Can you work these out from the model? Positions are in its coordinate system, mm. Face numbers are marked on the shaded views. A direction names the side the tool comes from. Give positions to 0.01 mm unless a question says otherwise; leave off trailing zeros. Order: outer loops, then holes, each group sorted by start corner. A loop starts at its lowest first (then second) coordinate and runs counter-clockwise, first axis right, second up. Notation, with made-up numbers: (32, -32) - (62, -32) arc R11 cw to (62, -28) - close; hole circle Ø4 at (58, -7). An arc over 180 degrees is marked (long way). Answer as a JSON object with one key per item and string values.
```python
from build123d import *

# Parameters (mm, degrees)
F0_W     = 84.4102278352
F0_H     = 68.1378934532
F0_R     = 12.3215660832
F1_DEPTH = 30.734
F2_R     = 13.2353706436
F3_DEPTH = 96.012
F2_R_2   = 9.0233824653
F4_DEPTH = 53.34
F2_R_3   = 4.6999449214
F5_DEPTH = 26.416


with BuildPart() as f1:
    # F0 (on Front) → F1 (new body)
    with BuildSketch(Plane.XZ):
        with Locations((0.754147768, -7.0776222274)):
            Rectangle(F0_W, F0_H)
        Circle(F0_R, mode=Mode.SUBTRACT)
    extrude(amount=F1_DEPTH)

    # F2 (on face) → F3 (join)
    with BuildSketch(Plane.XY.offset(26.9913244992)):
        with Locations((-12.7083817497, -14.5293129608)):
            Circle(F2_R)
    extrude(amount=F3_DEPTH)

    # F2 (on face) → F4 (join)
    with BuildSketch(Plane.XY.offset(26.9913244992)):
        with Locations((9.9861975759, -14.3468007445)):
            Circle(F2_R_2)
    extrude(amount=F4_DEPTH)

    # F2 (on face) → F5 (join)
    with BuildSketch(Plane.XY.offset(26.9913244992)):
        with Locations((-34.5160663128, -12.256086804)):
            Circle(F2_R_3)
    extrude(amount=F5_DEPTH)


solid = f1.part
```
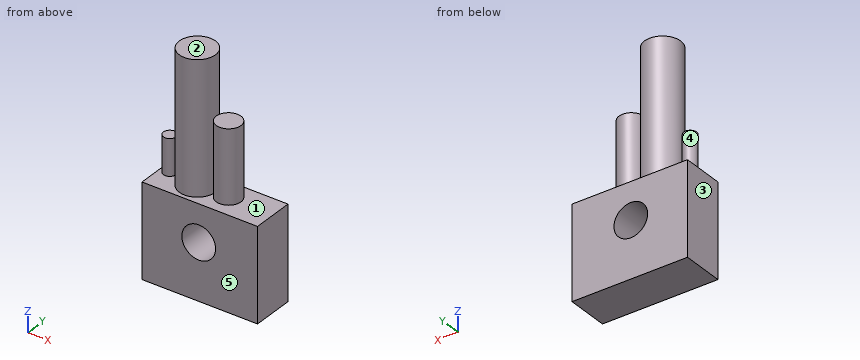
Q1. I'm going to push flat-ended pins straight in: pin 1 Ø12 at (x, y) = (16, -20) entering from +Z; pin 2 Ø10.5 at (x, y) = (-33.5, -13) entering from +Z; pin 3 Ø3 at (x, z) = (-3, 97) entering from -Y. Where does each tip first touch, or does it pass through?
Recorded:
{"pin 1": "stops at z = 80.33", "pin 2": "stops at z = 53.41", "pin 3": "stops at y = -24.91"}
Q2. I need wall thicknesses on L1, parallel to Z at x = 0, y = -10; L2, parallel to Z at x = 0, y = -11; L3, parallel to Z at x = -28, y = -22.5. Which ranges of each line are inside material? Lowest first, please.
Recorded:
{"L1": "z = -41.15 to -12.32, 12.32 to 26.99", "L2": "z = -41.15 to -12.32, 12.32 to 123", "L3": "z = -41.15 to 26.99"}
Q3. Which directions (+Z, -Z, +X, -X, +Y, -Y) give clear straight access to the entire face, cutting with the end or side of a thin tool? Please do the marked faces 1 and 2.
Recorded:
{"face 1": "+Z", "face 2": "+Z, +X, -X, +Y, -Y"}
Q4. If we section it at D-D, the plane x = 29.5: Please give me the cut outline in (y, z).
Recorded:
{"outline": "(-30.73, -41.15) - (0, -41.15) - (0, 26.99) - (-30.73, 26.99) - close"}
Q5. We'd pull the mould along X, two halves only. Please class the marked faces 3, 4 and 5: released by +X, released by -X, zero draft, split by the parting line, or undercut.
Recorded:
{"face 3": "released by -X", "face 4": "undercut", "face 5": "zero draft"}
Q6. If we section it at C-C, the plane y = -21.5: Please give me the cut outline in (x, z).
Recorded:
{"outline": "(-41.45, -41.15) - (42.96, -41.15) - (42.96, 26.99) - (15.49, 26.99) - (15.49, 80.33) - (4.49, 80.33) - (4.49, 26.99) - (-1.46, 26.99) - (-1.46, 123) - (-23.96, 123) - (-23.96, 26.99) - (-41.45, 26.99) - close; hole circle Ø24.64 at (0, 0)"}
Q7. If we section it at A-A, the plane z = 0: Please give me the cut outline in (x, y), then the cut area to 3 significant figures.
Recorded:
{"outline": "(-41.45, -30.73) - (-12.32, -30.73) - (-12.32, 0) - (-41.45, 0) - close; (12.32, -30.73) - (42.96, -30.73) - (42.96, 0) - (12.32, 0) - close", "area": "1,840 mm^2"}
Q8. If we section it at B-B, the plane x = 8.5: Please give me the cut outline in (y, z).
Recorded:
{"outline": "(-30.73, -41.15) - (0, -41.15) - (0, -8.92) - (-30.73, -8.92) - close; (-30.73, 8.92) - (0, 8.92) - (0, 26.99) - (-5.45, 26.99) - (-5.45, 80.33) - (-23.25, 80.33) - (-23.25, 26.99) - (-30.73, 26.99) - close"}
